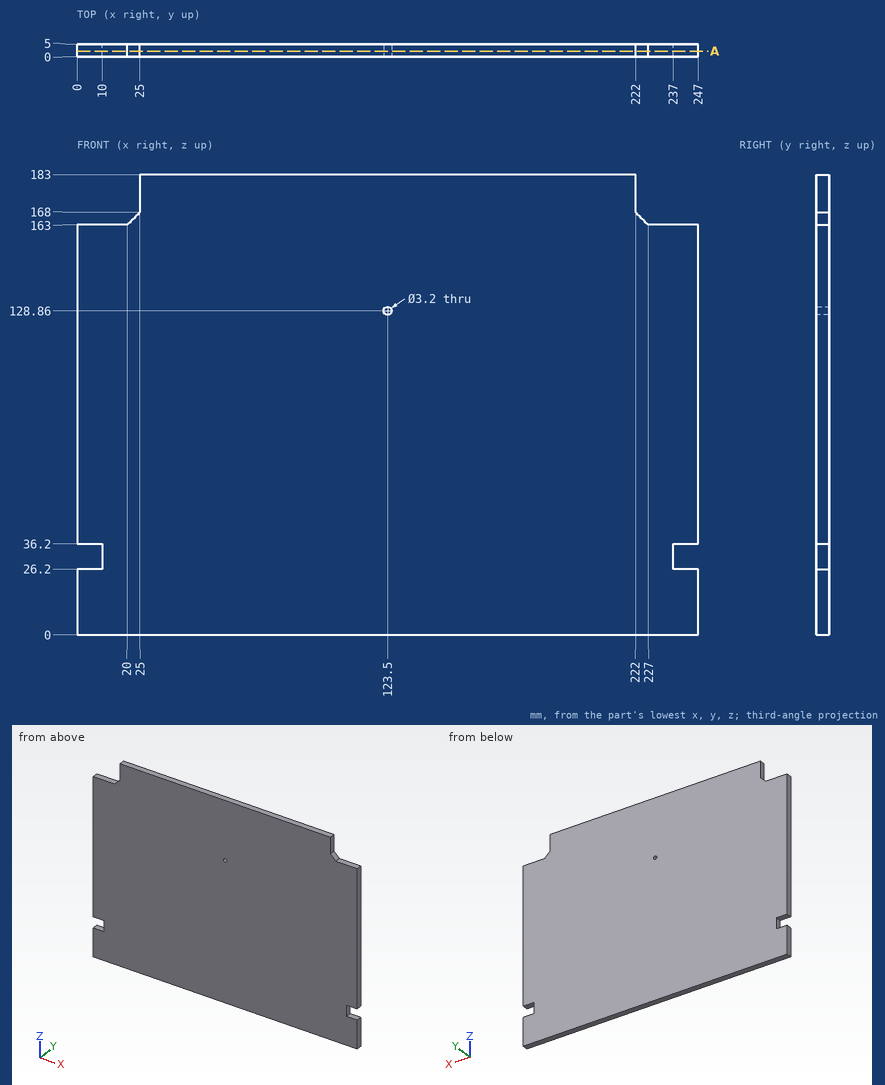
Check sheet for the drawn part. Datum: minimum x, y, z corner. Units: mm. Round coordinates to 2 decimals unless told otherwise and drop trailing zeros. Write each loop counter-clockwise with the first axis right and the second up, starting at its lowest first coordinate (ties: lowest second). Pieces come first, ordered by that corner, then holes. Notation, with made-up numbers: (29, 39.5) -> (48, 39.5) arc R17 cw to (48, 58.5) -> close; hole circle Ø1 at (51.25, 86.5). An arc over 180 degrees is marked (long way). One line per item, written item: value. Start each with the question number.
(1) Go/stop test with flat-tipped pins: pin 1 Ø1.5 at (x, y) = (4, 3.5) entering from +Z; pin 2 Ø2.5 at (y, z) = (2, 173) entering from -X; pin 3 Ø1.5 at (y, z) = (3.5, 33) entering from -X. Record where each tip stops, or that it passes through.
(2) Cross-section at A-A, the plane y = 2.15. Record the cut outline in (x, z).
(3) Scan lines: line 1 (Z direction, x = 123.5, y = 3.7); line 2 (X direction, y = 2.5, z = 128.86); line 3 (Z direction, x = 17.5, y = 0.3). Record each from-to range of solid material in increasing order. Write a range as [from, to].
Answer:
1. pin 1: z = 163
1. pin 2: x = 25
1. pin 3: x = 10
2. outline: (0, 0) -> (247, 0) -> (247, 26.2) -> (237, 26.2) -> (237, 36.2) -> (247, 36.2) -> (247, 163) -> (227, 163) -> (222, 168) -> (222, 183) -> (25, 183) -> (25, 168) -> (20, 163) -> (0, 163) -> (0, 36.2) -> (10, 36.2) -> (10, 26.2) -> (0, 26.2) -> close; hole circle Ø3.2 at (123.5, 128.86)
3. line 1: [0, 127.26], [130.46, 183]
3. line 2: [0, 121.9], [125.1, 247]
3. line 3: [0, 163]
